Autodesk Inventor part; units mm, degrees
ref_plane "YZ Plane" through (0, 0, 0) normal (1, 0, 0) x (0, 1, 0)
ref_plane "XZ Plane" through (0, 0, 0) normal (0, 1, 0) x (-1, 0, 0)
ref_plane "XY Plane" through (0, 0, 0) normal (0, 0, 1) x (1, 0, 0)
sketch "Skizze1" plane through (0, 0, 0) normal (0, 1, 0) x (-1, 0, 0)
  line L0 (-2, 0) -> (-161.05, 0)
  line L1 (-163.05, -2) -> (-163.05, -18)
  line L2 (-161.05, -20) -> (-2, -20)
  line L3 (0, -18) -> (0, -2)
  circle A0 centre (-154.05, -10) radius 3.05
  line L4 (0, -10) -> (-163.05, -10) construction
  line L5 (-163.05, -20) -> (-164.05, -20) construction
  line L6 (-164.05, -20) -> (-164.05, -1) construction
  line L7 (-164.05, -1) -> (-163.05, -1) construction
  line L8 (-163.05, -1) -> (-163.05, -20) construction
  line L9 (-164.05, -20) -> (-169.05, -20) construction
  line L10 (-169.05, -20) -> (-169.05, -1) construction
  line L11 (-169.05, -1) -> (-164.05, -1) construction
  line L12 (-164.05, -1) -> (-164.05, -20) construction
  circle A1 centre (-10, -10) radius 3.05
  line L13 (-13.05, -20) -> (-13.05, 0) construction
  arc A2 (-2, -20) -> (0, -18) centre (-2, -18) ccw
  arc A3 (0, -2) -> (-2, 0) centre (-2, -2) ccw
  arc A4 (-163.05, -18) -> (-161.05, -20) centre (-161.05, -18) ccw
  arc A5 (-161.05, 0) -> (-163.05, -2) centre (-161.05, -2) ccw
  point P0 (0, 0)
  point P1 (0, -20)
  dimension "d0" = 20
  dimension "d2" = 5
  dimension "d3" = 1
  dimension "d5" = 10
  dimension "d6" = 6.1
  dimension "d7" = 156
  dimension "d8" = 10
  dimension "d9" = 6.1
  dimension "d10" = 2
extrude "Extrusion1" add sketch "Skizze1" along normal blind 5
properties part number "Slider_Winkel_Abstandshalter"
Design review of the part built by this model. Coordinates are the model's own, in mm. Coordinates: 2 decimals unless noted, no trailing zeros. Loops run counter-clockwise (first coordinate to the right, second up) from the corner with the lowest first, then second, coordinate; pieces in that order, holes last. Notation, with made-up numbers: M -28.5,82 L 11.5,82 A25 ccw 11.5,94 Z; hole C 42.5,-4.75 d10. An arc over 180 degrees is marked long. Use one line per item in the form item = value.
(1) For line 1 along X through (y, z) = (4.75, -9.75); line 2 along X through (y, z) = (3, -8.75); line 3 along Z through (x, y) = (154.05, 2), list the stretches that pass through material, from the lowest coordinate up. Write a range as from..to.
Return value:
line_1 = 0..6.96, 13.04..151.01, 157.09..163.05
line_2 = 0..7.22, 12.78..151.27, 156.83..163.05
line_3 = -20..-13.05, -6.95..0
(2) Consider section C-C (z = -10). Write out the cut boundary in (x, y), and give its area (3 significant figures).
Return value:
outline = M 0,0 L 6.95,0 L 6.95,5 L 0,5 Z; M 13.05,0 L 151,0 L 151,5 L 13.05,5 Z; M 157.1,0 L 163.05,0 L 163.05,5 L 157.1,5 Z
area = 754 mm2
(3) Draft analysis for pull direction X (two halves, no side actions). For faces 1 (the face through (163.05, 2, -10)), 2 (the face through (157.1, 2.5, -10.1)), 3 (the face through (80, 2, 0)), 4 (the face through (0, 2, -10)), state which applies: pulls with the +X half, pulls with the -X half, needs draft (parallel to the pull), parting line crosses it, or undercut.
Return value:
face_1 = pulls with the +X half
face_2 = undercut
face_3 = needs draft
face_4 = pulls with the -X half
(4) Clearance check with a flat-ended pin moving along its axis: P1, Ø6, axis at x = 109, z = -8, coming from the -Y side. State where the tip first meets the part, or that it passes through.
Return value:
P1 = 0
(5) Consider section A-A (x = 154.05). Write out the cut boundary in (y, z), and give its area (3 significant figures).
Return value:
outline = M 0,-20 L 5,-20 L 5,-13.05 L 0,-13.05 Z; M 0,-6.95 L 5,-6.95 L 5,0 L 0,0 Z
area = 69.5 mm2
(6) Consider section B-B (y = 3.4). Write out the cut boundary in (x, z), and give its area (3 significant figures).
Return value:
outline = M 0,-18 A2 ccw 2,-20 L 161.05,-20 A2 ccw 163.05,-18 L 163.05,-2 A2 ccw 161.05,0 L 2,0 A2 ccw 0,-2 Z; hole C 10,-10 d6.1; hole C 154.05,-10 d6.1
area = 3,200 mm2
